Geometry: see drawing. Coordinates: mm, zero at the bounding-box minimum. Give positions to 0.01 mm unless a question says otherwise; leave off trailing zeros. Loops run counter-clockwise (first coordinate to the right, second up) from the corner with the lowest first, then second, coordinate; pieces in that order, holes last. Notation, with made-up numbers: M 36.25,11 L 76.25,11 A24 cw 76.25,30 Z; hole C -8,84.5 d2. An arc over 180 degrees is marked long. Put each result on its own line as item: value.
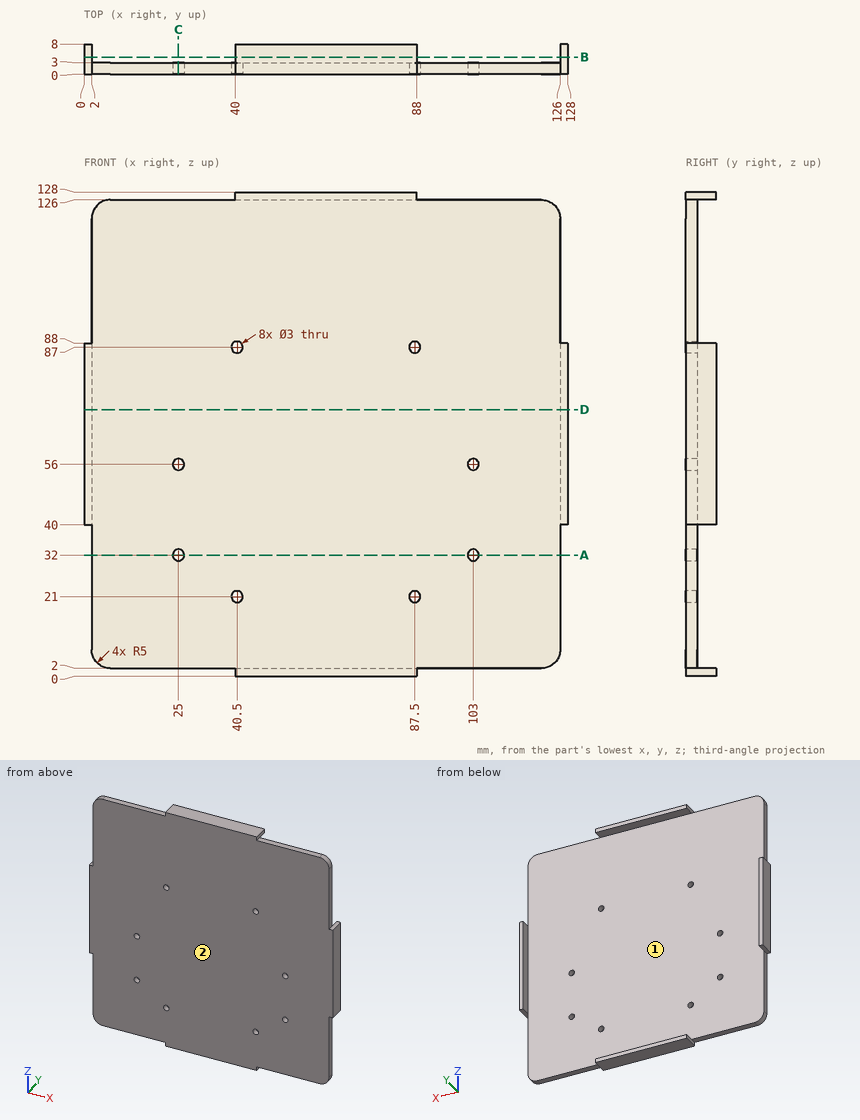
1. Section query D-D (z = 70.5). Output: boundary loops of the cut face in (x, y).
Found:
outline: M 0,0 L 128,0 L 128,8 L 126,8 L 126,3 L 2,3 L 2,8 L 0,8 Z
2. Section query B-B (y = 4.5). Output: boundary loops of the cut face in (x, z).
Found:
outline: M 0,40 L 2,40 L 2,88 L 0,88 Z; M 40,0 L 88,0 L 88,2 L 40,2 Z; M 40,126 L 88,126 L 88,128 L 40,128 Z; M 126,40 L 128,40 L 128,88 L 126,88 Z
3. Section query C-C (x = 25). Output: boundary loops of the cut face in (y, z).
Found:
outline: M 0,2 L 3,2 L 3,30.5 L 0,30.5 Z; M 0,33.5 L 3,33.5 L 3,54.5 L 0,54.5 Z; M 0,57.5 L 3,57.5 L 3,126 L 0,126 Z
4. Contact query for flat-ended pins moving along their axis: P1, Ø3.5, axis at x = 106.5, y = 1, coming from the +Z side; P2, Ø0.6, axis at x = 1, y = 3.5, coming from the +Z side; P3, Ø1, axis at y = 3, z = 127, coming from the +X side. Output: stop coordinate, or through.
Found:
P1: z = 126
P2: z = 88
P3: x = 88
5. Material intervals for line 1 (X direction, y = 2.75, z = 56); line 2 (Z direction, x = 103, y = 0.9); line 3 (X direction, y = 1.6, z = 87), sorted ascending. Write a range as from..to.
Found:
line 1: 0..23.5, 26.5..101.5, 104.5..128
line 2: 2..30.5, 33.5..54.5, 57.5..126
line 3: 0..39, 42..86, 89..128
6. Draft query along Z for the marked faces 1 and 2. Return one class per face: pulls with the +Z half, pulls with the -Z half, needs draft (parallel to the pull), parting line crosses it, or undercut.
Found:
face 1: undercut
face 2: needs draft
7. Section query A-A (z = 32). Output: boundary loops of the cut face in (x, y), plus the area to 3 significant figures.
Found:
outline: M 2,0 L 23.5,0 L 23.5,3 L 2,3 Z; M 26.5,0 L 101.5,0 L 101.5,3 L 26.5,3 Z; M 104.5,0 L 126,0 L 126,3 L 104.5,3 Z
area: 354 mm^2
